Read the model definition and answer for the solid it produces. Units are mm, in the model's axes. A direction names the side the tool comes from. Coordinates: 2 decimals unless noted, no trailing zeros. Loops run counter-clockwise (first coordinate to the right, second up) from the corner with the lowest first, then second, coordinate; pieces in that order, holes last. Notation, with made-up numbers: (85, 38.25) -> (140, 38.25) arc R11 ccw to (140, 48.25) -> close; hole circle Ø6 at (47.25, -23). An arc over 180 degrees is marked (long way). Answer as a JSON object with one key per item and string values. Group by question number.
Q1. Straight lines are drawn through the part: line 1 along Z through (x, y) = (-2.5, -1); line 2 along Z through (x, y) = (-11.5, 2); line 3 along X through (y, z) = (1.5, -28). For each, find the intervals that lie inside material, in ascending order. Write a range as [from, to].
Q2. For faces 5 (the flat face through (26.095, 0, -14)), 6 (the flat face through (0, 0, 1)), 7 (the flat face through (-1.8, 6, -2.9)), determine the directions among +Z, -Z, +X, -X, +Y, -Y from which every point of the face is accessible in a straight line to the end or side of a thin tool.
Q3. The part is cut by section A-A on x = 0. Write down the section's boundary in (y, z).
Q4. Each of these flat-tipped pins is pushed along its axis until it touches: P1, Ø2.5, axis at y = 0, z = -18, coming from the +X side; P2, Ø1.6, axis at y = 0, z = -18, coming from the -X side; P3, Ø3, axis at y = 0, z = -18, coming from the -X side; P4, Ø9.5, axis at x = 3, y = 0, coming from the +Z side. Where does it stop, or does it pass through?
Q5. The part is cut by section D-D on y = 7. Write down the section's boundary in (x, z), and give its area (3 significant figures).
Q6. Determine the mould class of faces 1 (the flat face through (0, 0, 0)), 2 (the cylindrical face through (-5.961, -26.846, 4.437)), 3 (the cylindrical face through (-3.47, -15.62, 4.94)), 4 (the flat face through (-1.8, -6, -2.9)) for opening direction Y: released by +Y, released by -Y, zero draft, split by the parting line, or undercut.
Q7. The part is cut by section B-B on z = -18. State how many separate pieces and enclosed holes the cut face has, and give its area (3 significant figures).
from build123d import *

# Parameters (mm, degrees)
SKETCH1_R                = 27.5
BOSS_EXTRUDE1_DEPTH      = 1
SKETCH2_R                = 27.5
SKETCH2_R_2              = 16
BOSS_EXTRUDE2_DEPTH      = 8
SKETCH3_W                = 1.095229805
SKETCH3_H                = 12
BOSS_EXTRUDE3_DEPTH      = 28
BOSS_EXTRUDE4_DEPTH      = 6
BOSS_EXTRUDE4_DEPTH_BACK = 6
CUT_EXTRUDE1_DEPTH       = 67.624274012
CUT_EXTRUDE1_DEPTH_BACK  = 67.624274012
SKETCH4_R                = 1


with BuildPart() as part:
    # Sketch1 → Boss-Extrude1 (new body)
    with BuildSketch(Plane.XY):
        Circle(SKETCH1_R)
    extrude(amount=BOSS_EXTRUDE1_DEPTH)

    # Sketch2 → Boss-Extrude2 (add)
    with BuildSketch(Plane.XY.offset(1)):
        Circle(SKETCH2_R)
        Circle(SKETCH2_R_2, mode=Mode.SUBTRACT)
    extrude(amount=BOSS_EXTRUDE2_DEPTH)

    # Sketch3 → Boss-Extrude3 (add)
    with BuildSketch(Plane(origin=(0, 0, 0), x_dir=(-1, 0, 0), z_dir=(0, 0, -1))):
        with Locations((-25.547614903, 0)):
            Rectangle(SKETCH3_W, SKETCH3_H)
        with Locations((25.547614903, 0)):
            Rectangle(SKETCH3_W, SKETCH3_H)
    extrude(amount=BOSS_EXTRUDE3_DEPTH)

    # Sketch6 → Boss-Extrude4 (add, two sides: drawn at the far end of the back side and taken through both)
    with BuildSketch(Plane(origin=(0, 0, 0), x_dir=(1, 0, 0), z_dir=(0, 1, 0)).offset(-BOSS_EXTRUDE4_DEPTH_BACK)):
        with BuildLine():
            ThreePointArc((-26.095229805, 28), (0, 54.095229805), (26.095229805, 28))
            ThreePointArc((26.095229805, 28), (0, 1.904770195), (-26.095229805, 28))
        make_face()
        with BuildLine():
            ThreePointArc((-25, 28), (0, 53), (25, 28))
            ThreePointArc((25, 28), (0, 3), (-25, 28))
        make_face(mode=Mode.SUBTRACT)
    extrude(amount=BOSS_EXTRUDE4_DEPTH + BOSS_EXTRUDE4_DEPTH_BACK)

    # Sketch4 → Cut-Extrude1 (cut, two sides: drawn at the far end of the back side and taken through both)
    with BuildSketch(Plane(origin=(0, 0, 0), x_dir=(0, 0, -1), z_dir=(1, 0, 0)).offset(-CUT_EXTRUDE1_DEPTH_BACK)):
        with Locations((18, 0)):
            Circle(SKETCH4_R)
    extrude(amount=CUT_EXTRUDE1_DEPTH + CUT_EXTRUDE1_DEPTH_BACK, mode=Mode.SUBTRACT)


solid = part.part
Final values:
{
 "1": {"line 1": "z = [-53.98, -52.87], [-3.13, -2.02], [0, 1]", "line 2": "z = [-51.42, -50.2], [-5.8, -4.58], [0, 1]", "line 3": "x = [-26.1, -25], [25, 26.1]"},
 "2": {"face 5": "-Z, +X, +Y, -Y", "face 6": "+Z", "face 7": "-Z, +X, -X, +Y"},
 "3": {"outline": "(-27.5, 0) -> (27.5, 0) -> (27.5, 9) -> (16, 9) -> (16, 1) -> (-16, 1) -> (-16, 9) -> (-27.5, 9) -> close; (-6, -54.1) -> (6, -54.1) -> (6, -53) -> (-6, -53) -> close; (-6, -3) -> (6, -3) -> (6, -1.9) -> (-6, -1.9) -> close"},
 "4": {"P1": "stops at x = 26.1", "P2": "passes through", "P3": "stops at x = -26.1", "P4": "stops at z = 1"},
 "5": {"outline": "(-26.59, 0) -> (26.59, 0) -> (26.59, 9) -> (14.39, 9) -> (14.39, 1) -> (-14.39, 1) -> (-14.39, 9) -> (-26.59, 9) -> close", "area": "248 mm2"},
 "6": {"face 1": "zero draft", "face 2": "split by the parting line", "face 3": "undercut", "face 4": "released by -Y"},
 "7": {"separate pieces": "8", "enclosed holes": "0", "area": "45.7 mm2"}
}
